```python
from build123d import *

# Parameters (mm, degrees)
F0_W     = 50.8
F0_H     = 38.1
F1_DEPTH = 76.2
F2_R     = 17.4803225392
F3_DEPTH = 38.101
F4_R     = 5.08


with BuildPart() as f1:
    # F0 (on Top) → F1 (new body)
    with BuildSketch(Plane.XY):
        with Locations((-25.4, -6.35)):
            Rectangle(F0_W, F0_H)
    extrude(amount=F1_DEPTH)

    # F2 (on face) → F3 (cut, through all)
    with BuildSketch(Plane.XZ.offset(25.4)):
        with BuildLine():
            ThreePointArc((-38.4466977771, 16.2261378818), (-36.2780752576, 20.4825429519), (-35.530821321, 25.2007544041))
            ThreePointArc((-35.530821321, 25.2007544041), (-35.5426781239, 25.802374467), (-35.5782301185, 26.4030601914))
            ThreePointArc((-35.5782301185, 26.4030601914), (-38.3981973117, 21.7051818884), (-38.4466977771, 16.2261378818))
        make_face()
        with BuildLine():
            ThreePointArc((-35.5782301185, 26.4030601914), (-35.5426781239, 25.802374467), (-35.530821321, 25.2007544041))
            ThreePointArc((-35.530821321, 25.2007544041), (-36.2780752576, 20.4825429519), (-38.4466977771, 16.2261378818))
            ThreePointArc((-38.4466977771, 16.2261378818), (-30.7853938644, 8.7355753596), (-20.5657055583, 11.9545931397))
            ThreePointArc((-20.5657055583, 11.9545931397), (-21.3730987717, 17.05320374), (-18.1779448175, 21.1076710371))
            ThreePointArc((-18.1779448175, 21.1076710371), (-25.3272484905, 28.8513160491), (-35.5782301185, 26.4030601914))
        make_face()
        with BuildLine():
            ThreePointArc((-38.4466977771, 16.2261378818), (-38.3981973117, 21.7051818884), (-35.5782301185, 26.4030601914))
            ThreePointArc((-35.5782301185, 26.4030601914), (-65.4965501841, 29.3431245248), (-38.4466977771, 16.2261378818))
        make_face()
        with BuildLine():
            ThreePointArc((-8.6975224724, 15.4270771891), (-11.8284701462, 20.9530964233), (-18.1779448175, 21.1076710371))
            ThreePointArc((-18.1779448175, 21.1076710371), (-17.9969955306, 19.9986578535), (-17.9364446703, 18.8766121864))
            ThreePointArc((-17.9364446703, 18.8766121864), (-18.6158988239, 15.1743371933), (-20.5657055583, 11.9545931397))
            ThreePointArc((-20.5657055583, 11.9545931397), (-13.3305831879, 9.2441993148), (-8.6975224724, 15.4270771891))
        make_face()
        with BuildLine():
            ThreePointArc((-17.9364446703, 18.8766121864), (-17.9969955306, 19.9986578535), (-18.1779448175, 21.1076710371))
            ThreePointArc((-18.1779448175, 21.1076710371), (-21.3730987717, 17.05320374), (-20.5657055583, 11.9545931397))
            ThreePointArc((-20.5657055583, 11.9545931397), (-18.6158988239, 15.1743371933), (-17.9364446703, 18.8766121864))
        make_face()
        with Locations((0, 57.3963969946)):
            Circle(F2_R)
    extrude(amount=-F3_DEPTH, mode=Mode.SUBTRACT)

    # F4
    f4_edges = [f1.edges().sort_by_distance(p)[0] for p in [
        (-17.480323, 12.7, 57.396397),
    ]]
    fillet(f4_edges, radius=F4_R)


solid = f1.part
```
Geometry check sheet. Reference: the model listing, model coordinates, mm. A direction names the side the tool comes from. Round coordinates to 2 decimals unless told otherwise and drop trailing zeros. Write each loop counter-clockwise with the first axis right and the second up, starting at its lowest first coordinate (ties: lowest second). Pieces come first, ordered by that corner, then holes. Notation, with made-up numbers: (72, 79.25) -> (87, 79.25) arc R15 cw to (87, 104.25) -> close; hole circle Ø9 at (-5, -17.5). An arc over 180 degrees is marked (long way). Put each result on its own line as item: value.
1) Thickness scan on probe 1 along Z at (x, y) = (-28, 9.5); probe 2 along Z at (x, y) = (-11.5, -9.5); probe 3 along Z at (x, y) = (-15, 11). Record the ranges inside material, lowest first. Write a range as from..to.
Recorded:
probe 1: z = 0..8.46, 29.3..76.2
probe 2: z = 0..10.11, 20.74..44.23, 70.56..76.2
probe 3: z = 0..8.99, 21.87..46.12, 68.68..76.2
2) Access from +Z, -Z, +X, -X, +Y, -Y to the whole of each face (thin tool, end or side, straight path). Record for faces 1 (the face through (-43.96, -6.62, 11.55)), 2 (the face through (-30.938, -6.617, 8.773)), 3 (the face through (-26, -25.4, 38)).
Recorded:
face 1: -X, +Y, -Y
face 2: +Y, -Y
face 3: +Z, -Z, +X, -X, -Y
3) Depth check by flat-ended pin: P1, Ø1, axis at x = -8, z = 37, coming from the +Y side; P2, Ø12, axis at x = -14.5, z = 55, coming from the +Y side. Enter the tip coordinate at first touch or a pass-through.
Recorded:
P1: stops at y = 12.7
P2: stops at y = 12.35
4) Cross-section at A-A, the plane x = -29. Enter the section's corners in (y, z), plus the area to 3 significant figures.
Recorded:
outline: (-25.4, 0) -> (12.7, 0) -> (12.7, 8.47) -> (-25.4, 8.47) -> close; (-25.4, 29.28) -> (12.7, 29.28) -> (12.7, 76.2) -> (-25.4, 76.2) -> close
area: 2,110 mm2
5) Cross-section at C-C, the plane x = -40. Enter the section's corners in (y, z).
Recorded:
outline: (-25.4, 0) -> (12.7, 0) -> (12.7, 14.41) -> (-25.4, 14.41) -> close; (-25.4, 35.99) -> (12.7, 35.99) -> (12.7, 76.2) -> (-25.4, 76.2) -> close
6) Cross-section at B-B, the plane y = -6. Enter the section's corners in (x, z).
Recorded:
outline: (-50.8, 0) -> (0, 0) -> (0, 39.92) arc R17.48 cw to (0, 74.88) -> (0, 76.2) -> (-50.8, 76.2) -> (-50.8, 40.47) arc R15.27 cw to (-35.58, 26.4) arc R10.43 cw to (-18.18, 21.11) arc R6.44 cw (long way) to (-20.57, 11.95) arc R10.43 cw to (-38.45, 16.23) arc R15.27 cw to (-50.8, 9.93) -> close
7) Release check for a two-part mould opening along Z. For faces 4 (the face through (-50.8, -7, 58)), 5 (the face through (-25.18, -6.617, 28.805)), 6 (the face through (-26, -6, 76.2)) record: pulls with the +Z half, pulls with the -Z half, needs draft (parallel to the pull), parting line crosses it, or undercut.
Recorded:
face 4: needs draft
face 5: undercut
face 6: pulls with the +Z half
